Verification items for this drawing (mm, ordinates from the low corner). A direction names the side the tool comes from. Coordinates: 2 decimals unless noted, no trailing zeros. Order: outer loops, then holes, each group sorted by start corner. A loop starts at its lowest first (then second) coordinate and runs counter-clockwise, first axis right, second up. Notation, with made-up numbers: M 53.25,14.25 L 82.25,14.25 A13 ccw 82.25,37.25 Z; hole C 38,28 d8. An arc over 180 degrees is marked long. Use CSV: the item, a comma, the result in double quotes. Start each with the question number.
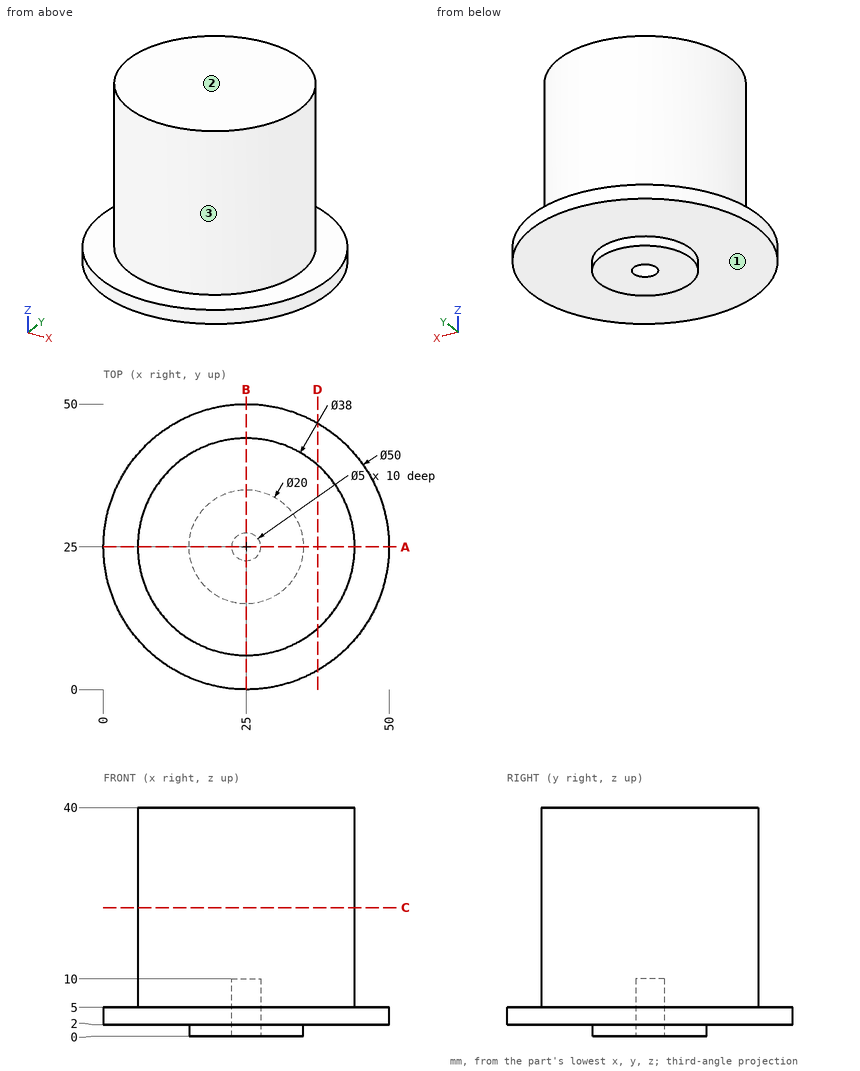
1) Section check D-D on x = 37.5. Record the boundary of the cut face in (y, z).
2) Set-up check for the marked faces 1, 2 and 3: record each of +Z, -Z, +X, -X, +Y, -Y from which the full face is reachable in a straight line by a thin tool's end or side.
3) Material ranges on line 1 along Y through (x, z) = (25, 2.25); line 2 along Y through (x, z) = (25, 6.25); line 3 along Z through (x, y) = (8, 18), recorded low to high.
4) Section check A-A on y = 25. Record the boundary of the cut face in (x, z).
5) Gauge pin test, flat ends, axial feed: P1, Ø1.5, axis at x = 24, y = 25, coming from the -Z side; P2, Ø4, axis at x = 8.5, z = 21, coming from the +Y side; P3, Ø1, axis at x = 16.5, y = 14, coming from the -Z side; P4, Ø1, axis at x = 5.5, y = 8, coming from the +Z side. Record the tip position at first contact, or that the pin passes through.
6) Section check C-C on z = 22.5. Record the boundary of the cut face in (x, y), then the cut area to 3 significant figures.
Results are:
1,outline,"M 3.35,2 L 46.65,2 L 46.65,5 L 39.31,5 L 39.31,40 L 10.69,40 L 10.69,5 L 3.35,5 Z"
2,face 1,"-Z"
2,face 2,"+Z, +X, -X, +Y, -Y"
2,face 3,"+Z"
3,line 1,"y = 0 to 22.5, 27.5 to 50"
3,line 2,"y = 6 to 22.5, 27.5 to 44"
3,line 3,"z = 2 to 40"
4,outline,"M 0,2 L 15,2 L 15,0 L 22.5,0 L 22.5,10 L 27.5,10 L 27.5,0 L 35,0 L 35,2 L 50,2 L 50,5 L 44,5 L 44,40 L 6,40 L 6,5 L 0,5 Z"
5,P1,"stops at z = 10"
5,P2,"stops at y = 37.28"
5,P3,"stops at z = 2"
5,P4,"passes through"
6,outline,"C 25,25 d38"
6,area,"1,130 mm²"
